CAD build for the part. Positions are in the model's coordinates, mm. A direction names the side the tool comes from. Round coordinates to 2 decimals unless told otherwise and drop trailing zeros. Loops run counter-clockwise (first coordinate to the right, second up) from the corner with the lowest first, then second, coordinate; pieces in that order, holes last. Notation, with made-up numbers: (23.5, -7) - (55.5, -7) arc R23 cw to (55.5, 14) - close; hole circle Ø6 at (13.25, 70.5). An arc over 180 degrees is marked (long way). One line per question, with ' | ' between items.
```python
from build123d import *

# Parameters (mm, degrees)
SKETCH1_W           = 110
SKETCH1_H           = 80
BOSS_EXTRUDE1_DEPTH = 3
SKETCH1_3_W         = 116
SKETCH1_3_H         = 86
SKETCH1_3_W_2       = 110
SKETCH1_3_H_2       = 80
BOSS_EXTRUDE2_DEPTH = 53
SKETCH2_R           = 4.5
CUT_EXTRUDE1_DEPTH  = 53
SKETCH3_R           = 5.5
CUT_EXTRUDE2_DEPTH  = 53
SKETCH5_W           = 113
SKETCH5_H           = 35
CUT_EXTRUDE3_DEPTH  = 83
SKETCH6_R           = 5
BOSS_EXTRUDE3_DEPTH = 15
SKETCH8_R           = 1.75
CUT_EXTRUDE4_DEPTH  = 25
SKETCH9_R           = 3
CUT_EXTRUDE5_DEPTH  = 10
SKETCH10_R          = 5
SKETCH10_R_2        = 1.25
BOSS_EXTRUDE4_DEPTH = 50
SKETCH11_W          = 33.464657476
SKETCH11_H          = 24.968484897
CUT_EXTRUDE7_DEPTH  = 35


with BuildPart() as part:
    # Sketch1 → Boss-Extrude1 (new body)
    with BuildSketch(Plane(origin=(0, 0, 0), x_dir=(1, 0, 0), z_dir=(0, 1, 0))):
        with Locations((55, 40)):
            Rectangle(SKETCH1_W, SKETCH1_H)
    extrude(amount=BOSS_EXTRUDE1_DEPTH)

    # Sketch1<3> → Boss-Extrude2 (add)
    with BuildSketch(Plane(origin=(0, 0, 0), x_dir=(1, 0, 0), z_dir=(0, 1, 0))):
        with Locations((55, 40)):
            Rectangle(SKETCH1_3_W, SKETCH1_3_H)
        with Locations((55, 40)):
            Rectangle(SKETCH1_3_W_2, SKETCH1_3_H_2, mode=Mode.SUBTRACT)
    extrude(amount=BOSS_EXTRUDE2_DEPTH)

    # Sketch2 → Cut-Extrude1 (cut)
    with BuildSketch(Plane.ZY.offset(3)):
        with Locations((-7, 18)):
            Circle(SKETCH2_R)
    extrude(amount=-CUT_EXTRUDE1_DEPTH, mode=Mode.SUBTRACT)

    # Sketch3 → Cut-Extrude2 (cut)
    with BuildSketch(Plane(origin=(0, 0, -83), x_dir=(-1, 0, 0), z_dir=(0, 0, -1))):
        with Locations((-93, 18)):
            Circle(SKETCH3_R)
    extrude(amount=-CUT_EXTRUDE2_DEPTH, mode=Mode.SUBTRACT)

    # Sketch5 → Cut-Extrude3 (cut)
    with BuildSketch(Plane(origin=(0, 0, -83), x_dir=(-1, 0, 0), z_dir=(0, 0, -1))):
        with Locations((-53.5, 35.5)):
            Rectangle(SKETCH5_W, SKETCH5_H)
    extrude(amount=-CUT_EXTRUDE3_DEPTH, mode=Mode.SUBTRACT)

    # Sketch6 → Boss-Extrude3 (add)
    with BuildSketch(Plane(origin=(0, 3, 0), x_dir=(1, 0, 0), z_dir=(0, 1, 0))):
        with Locations((2, 78)):
            Circle(SKETCH6_R)
    extrude(amount=BOSS_EXTRUDE3_DEPTH)

    # Sketch8 → Cut-Extrude4 (cut)
    with BuildSketch(Plane(origin=(0, 18, 0), x_dir=(1, 0, 0), z_dir=(0, 1, 0))):
        with Locations((2, 78)):
            Circle(SKETCH8_R)
    extrude(amount=-CUT_EXTRUDE4_DEPTH, mode=Mode.SUBTRACT)

    # Sketch9 → Cut-Extrude5 (cut)
    with BuildSketch(Plane(origin=(0, 0, 0), x_dir=(-1, 0, 0), z_dir=(0, -1, 0))):
        with Locations((-2, 78)):
            Circle(SKETCH9_R)
    extrude(amount=-CUT_EXTRUDE5_DEPTH, mode=Mode.SUBTRACT)

    # Sketch10 → Boss-Extrude4 (add)
    with BuildSketch(Plane(origin=(0, 3, 0), x_dir=(1, 0, 0), z_dir=(0, 1, 0))):
        with Locations((108, 2)):
            Circle(SKETCH10_R)
        with Locations((108, 2)):
            Circle(SKETCH10_R_2, mode=Mode.SUBTRACT)
    extrude(amount=BOSS_EXTRUDE4_DEPTH)

    # Sketch11 → Cut-Extrude7 (cut)
    with BuildSketch(Plane(origin=(0, 3, 0), x_dir=(1, 0, 0), z_dir=(0, 1, 0))):
        with Locations((93.267671262, 12.484242449)):
            Rectangle(SKETCH11_W, SKETCH11_H)
    extrude(amount=CUT_EXTRUDE7_DEPTH, mode=Mode.SUBTRACT)


solid = part.part
```
(1) Cut at B-B, the plane y = 35. Write the cut outline in (x, z).
Results found:
outline: (-3, 0) - (110, 0) - (110, -83) - (113, -83) - (113, 3) - (-3, 3) - close
(2) Two-plate mould, pull along Z, no slides. Class faces 6 (the face through (-3, 13, -37)), 7 (the face through (59, 13, -83)), 8 (the face through (110, 28, -42)), 9 (the face through (0, 10, -78)): released by +Z, released by -Z, zero draft, split by the parting line, or undercut.
Results found:
face 6: zero draft | face 7: released by -Z | face 8: undercut | face 9: undercut
(3) Tool access for faces 1 (the face through (-1.5, 13.5, -7.1)), 2 (the face through (106, 38, -4)), 3 (the face through (2.65, 4.93, -75.07)), 4 (the face through (-1, 18, -1)), 5 (the face through (58, 10, -80)): list every direction of +Z, -Z, +X, -X, +Y, -Y with a clear straight run to the whole face (end or side of a thin tool).
Results found:
face 1: -X, +Y | face 2: -Z, -X | face 3: -Y | face 4: -Z, -X, +Y | face 5: +Y
(4) Drop flat-ended pins along their axis: P1, Ø10, axis at y = 41.5, z = -39.5, coming from the -X side; P2, Ø5.5, axis at x = 106.5, z = -2, coming from the -Y side; P3, Ø10, axis at x = 86.5, y = 32, coming from the -Z side; P4, Ø4, axis at x = 2, z = -78, coming from the -Y side. Give the stop position or say it passes through.
Results found:
P1: stops at x = 110 | P2: stops at y = 0 | P3: stops at z = 0 | P4: stops at y = 10
(5) Cut at D-D, the plane y = 42.5. Write the cut outline in (x, z).
Results found:
outline: (-3, 0) - (103.42, 0) arc R5 ccw to (110, -6.58) - (110, -83) - (113, -83) - (113, 3) - (-3, 3) - close; hole circle Ø2.5 at (108, -2)
(6) Cut at A-A, the plane x = 2. Write the cut outline in (y, z), then the cut area to 3 significant figures.
Results found:
outline: (0, -83) - (18, -83) - (18, -79.75) - (10, -79.75) - (10, -81) - (0, -81) - close; (0, -75) - (10, -75) - (10, -76.25) - (18, -76.25) - (18, -73) - (3, -73) - (3, 0) - (53, 0) - (53, 3) - (0, 3) - close | area: 470 mm²
(7) Cut at C-C, the plane z = -23.5. Write the cut outline in (x, y).
Results found:
outline: (-3, 0) - (113, 0) - (113, 53) - (110, 53) - (110, 3) - (0, 3) - (0, 18) - (-3, 18) - close
(8) Probe L1, parallel to Z at x = 2, y = 14; L2, parallel to X at y = 13.25, z = -78; L3, parallel to Z at x = 80, y = 16. List the from-to ranges inside material, lowest first.
Results found:
L1: z = -83 to -79.75, -76.25 to -73, 0 to 3 | L2: x = -3 to 0.25, 3.75 to 7, 110 to 113 | L3: z = -83 to -80, 0 to 3
